Autodesk Inventor part; units mm, degrees
ref_plane "YZ Plane" through (0, 0, 0) normal (1, 0, 0) x (0, 1, 0)
ref_plane "XZ Plane" through (0, 0, 0) normal (0, 1, 0) x (-1, 0, 0)
ref_plane "XY Plane" through (0, 0, 0) normal (0, 0, 1) x (1, 0, 0)
sketch "スケッチ1" plane through (0, 0, 0) normal (0, 1, 0) x (-1, 0, 0)
  circle A0 centre (0, 0) radius 5
  dimension "d0" = 10
extrude "押し出し1" add sketch "スケッチ1" along normal blind 51.8
sketch "スケッチ2" plane through (0, 51.8, 0) normal (0, 1, 0) x (1, 0, 0)
  circle A0 centre (0, 0) radius 4
  dimension "d3" = 8
extrude "押し出し2" add sketch "スケッチ2" along normal blind 51.6
sketch "スケッチ3" plane through (0, 0, 0) normal (0, -1, 0) x (1, 0, 0)
  circle A0 centre (0, 0) radius 5
  circle A1 centre (0, 0) radius 4
  dimension "d6" = 8
extrude "押し出し3" add sketch "スケッチ3" along normal blind 43 contours A1
properties part number "elbow_shaft3"
Model file for the job. Use its own axes, mm. A direction names the side the tool comes from. Round coordinates to 2 decimals unless told otherwise and drop trailing zeros. Write each loop counter-clockwise with the first axis right and the second up, starting at its lowest first coordinate (ties: lowest second). Pieces come first, ordered by that corner, then holes. Notation, with made-up numbers: M 6,-17 L 52,-17 A14 ccw 52,6 Z; hole C 67,26 d11. An arc over 180 degrees is marked long. Put each result on its own line as item: value.
Item 1: Probe L1, parallel to Y at x = -4.5, z = -0.75; L2, parallel to Z at x = 0.25, y = 29; L3, parallel to X at y = -32, z = 2.5. List the from-to ranges inside material, lowest first. Write a range as from..to.
Responses:
L1: 0..51.8
L2: -4.99..4.99
L3: -3.12..3.12
Item 2: Cut at A-A (z = 0). List the corners of the cut face in (x, y), and give its area (3 significant figures).
Responses:
outline: M -5,0 L -4,0 L -4,-43 L 4,-43 L 4,0 L 5,0 L 5,51.8 L 4,51.8 L 4,103.4 L -4,103.4 L -4,51.8 L -5,51.8 Z
area: 1,270 mm²
Item 3: Cut at B-B (x = 0). List the corners of the cut face in (y, z), and give its area (3 significant figures).
Responses:
outline: M -43,-4 L 0,-4 L 0,-5 L 51.8,-5 L 51.8,-4 L 103.4,-4 L 103.4,4 L 51.8,4 L 51.8,5 L 0,5 L 0,4 L -43,4 Z
area: 1,270 mm²
Item 4: Tool access for faces 1 (the cylindrical face through (-0.867, -21.199, 3.905)), 2 (the flat face through (0, 103.4, 0)), 3 (the cylindrical face through (-0.867, 77.239, -3.905)): list every direction of +Z, -Z, +X, -X, +Y, -Y with a clear straight run to the whole face (end or side of a thin tool).
Responses:
face 1: -Y
face 2: +Z, -Z, +X, -X, +Y
face 3: +Y
Item 5: Cut at D-D (y = 48.5). List the corners of the cut face in (x, z).
Responses:
outline: C 0,0 d10
Item 6: Cut at C-C (y = 85). List the corners of the cut face in (x, z).
Responses:
outline: C 0,0 d8
Item 7: Flat gauge pins, fed straight in: P1, Ø6, axis at x = 0.5, y = 55.5, coming from the +Z side; P2, Ø1.5, axis at y = 3, z = 1, coming from the -X side. Where does each tip first touch, or does it go through?
Responses:
P1: z = 4
P2: x = -4.99
